```python
from build123d import *

# Parameters (mm, degrees)
SKETCH2_R           = 1
BOSS_EXTRUDE1_DEPTH = 95
BOSS_EXTRUDE2_START = -12.5
SKETCH3_R           = 1.5
BOSS_EXTRUDE2_DEPTH = 1
BOSS_EXTRUDE3_START = -11.5
SKETCH4_R           = 1.5
BOSS_EXTRUDE3_DEPTH = 1


with BuildPart() as part:
    # Sketch2 → Boss-Extrude1 (new body)
    with BuildSketch(Plane.XY):
        Circle(SKETCH2_R)
    extrude(amount=-BOSS_EXTRUDE1_DEPTH)

    # Sketch3 → Boss-Extrude2 (add)
    with BuildSketch(Plane.XY.offset(BOSS_EXTRUDE2_START)):
        Circle(SKETCH3_R)
    extrude(amount=BOSS_EXTRUDE2_DEPTH)

    # Sketch4 → Boss-Extrude3 (add)
    with BuildSketch(Plane(origin=(0, 0, -95), x_dir=(-1, 0, 0), z_dir=(0, 0, -1)).offset(BOSS_EXTRUDE3_START)):
        with Locations(Location((0, 0, 0), (0, 0, 180))):
            Circle(SKETCH4_R)
    extrude(amount=-BOSS_EXTRUDE3_DEPTH)


solid = part.part
```
Model file for the job. Use its own axes, mm. A direction names the side the tool comes from. Coordinates: 2 decimals unless noted, no trailing zeros. Write each loop counter-clockwise with the first axis right and the second up, starting at its lowest first coordinate (ties: lowest second). Pieces come first, ordered by that corner, then holes. Notation, with made-up numbers: (74, 7) - (89, 7) arc R26 cw to (89, 43) - close; hole circle Ø6 at (26, -8.5). An arc over 180 degrees is marked (long way). Use a Markdown table: item, result. Add a question column.
Item 1: Band-saw the part on A-A, the plane x = 0. Write the cut outline in (y, z), and give its area (3 significant figures).
Item 2: Drop a flat-ended pin along its axis: pin 1 (1.5 mm diameter, centred on x = -0.5, y = 0.5, fed in from +Z). Give the stop position or say it passes through.
Item 3: 3-axis set-ups, long thin cutter, end or side, ignore diameter. For faces 1 (the face through (0, -1, -47)), 2 (the face through (0, -1, -6)), 3 (the face through (0, 0, -95)), 4 (the face through (0, -1, -89)): which of +Z, -Z, +X, -X, +Y, -Y reach the whole face in a straight line?
Item 4: Band-saw the part on B-B, the plane y = -0.5. Write the cut outline in (x, z).
Item 5: Drill centre lines: line 1 along Z through (x, y) = (0.8, 1.1); line 2 along Y through (x, z) = (-0.1, -16.5); line 3 along X through (y, z) = (0.6, -86.5). Where is each one in solid material? Low to high.
Item 6: Band-saw the part on C-C, the plane z = -75.5. Write the cut outline in (x, y).
A:
| question | item | result |
|---|---|---|
| 1 | outline | (-1.5, -83.5) - (-1, -83.5) - (-1, -95) - (1, -95) - (1, -83.5) - (1.5, -83.5) - (1.5, -82.5) - (1, -82.5) - (1, -12.5) - (1.5, -12.5) - (1.5, -11.5) - (1, -11.5) - (1, 0) - (-1, 0) - (-1, -11.5) - (-1.5, -11.5) - (-1.5, -12.5) - (-1, -12.5) - (-1, -82.5) - (-1.5, -82.5) - close |
| 1 | area | 192 mm² |
| 2 | pin 1 | stops at z = 0 |
| 3 | face 1 | none |
| 3 | face 2 | +Z |
| 3 | face 3 | -Z, +X, -X, +Y, -Y |
| 3 | face 4 | -Z |
| 4 | outline | (-1.41, -83.5) - (-0.87, -83.5) - (-0.87, -95) - (0.87, -95) - (0.87, -83.5) - (1.41, -83.5) - (1.41, -82.5) - (0.87, -82.5) - (0.87, -12.5) - (1.41, -12.5) - (1.41, -11.5) - (0.87, -11.5) - (0.87, 0) - (-0.87, 0) - (-0.87, -11.5) - (-1.41, -11.5) - (-1.41, -12.5) - (-0.87, -12.5) - (-0.87, -82.5) - (-1.41, -82.5) - close |
| 5 | line 1 | z = -83.5 to -82.5, -12.5 to -11.5 |
| 5 | line 2 | y = -0.99 to 0.99 |
| 5 | line 3 | x = -0.8 to 0.8 |
| 6 | outline | circle Ø2 at (0, 0) |
